CAD build for the part. Positions are in the model's coordinates, mm. Round coordinates to 2 decimals unless told otherwise and drop trailing zeros. Loops run counter-clockwise (first coordinate to the right, second up) from the corner with the lowest first, then second, coordinate; pieces in that order, holes last.
```python
from build123d import *
from build123d import SkipClean  # not in build123d's __all__

# Parameters (mm, degrees)
F0_W     = 14
F0_H     = 100
F0_R     = 1.64
F1_DEPTH = 1
F2_DEPTH = 10
F3_R     = 2
F4_DEPTH = 9.501


# Not quite as in the source:
# - after a boolean that leaves OpenCascade's solid faulty, fix() repairs it
# - a feature names something its author has since deleted; it is built from what else it names


with BuildPart() as f1:
    # F0 (on Front) → F1 (new body)
    with BuildSketch(Plane.XZ):
        Rectangle(F0_W, F0_H)
        with BuildLine():
            Line((-2.5, -44.5), (-2.5, -34.5))
            Line((-2.5, -34.5), (-0.8938540149, -34.5))
            ThreePointArc((-0.8938540149, -34.5), (-0.7822018331, -31.6835561779), (1.64, -33.125))
            ThreePointArc((1.64, -33.125), (1.4414438221, -33.9072018331), (0.8938540149, -34.5))
            Line((0.8938540149, -34.5), (2.5, -34.5))
            Line((2.5, -34.5), (2.5, -44.5))
            Line((2.5, -44.5), (0.8938540149, -44.5))
            ThreePointArc((0.8938540149, -44.5), (1.4414438221, -45.0927981669), (1.64, -45.875))
            ThreePointArc((1.64, -45.875), (-0.7822018331, -47.3164438221), (-0.8938540149, -44.5))
            Line((-0.8938540149, -44.5), (-2.5, -44.5))
        make_face(mode=Mode.SUBTRACT)
        Polygon((5, -21.096), (5, -29), (-5, -29), align=None, mode=Mode.SUBTRACT)
        Polygon((5, -19.096), (-5, -27), (-5, -11.192), align=None, mode=Mode.SUBTRACT)
        Polygon((5, -17.096), (-5, -9.192), (5, -1.288), align=None, mode=Mode.SUBTRACT)
        with Locations((-3.5, 45.167)):
            Circle(F0_R, mode=Mode.SUBTRACT)
        Polygon((-5, -7.19), (-5, 8.618), (5, 0.714), align=None, mode=Mode.SUBTRACT)
        Polygon((5, 18.522), (5, 2.714), (-5, 10.618), align=None, mode=Mode.SUBTRACT)
        Polygon((-5, 12.62), (-5, 28.428), (5, 20.524), align=None, mode=Mode.SUBTRACT)
        Polygon((5, 38.332), (5, 22.524), (-5, 30.428), align=None, mode=Mode.SUBTRACT)
        Polygon((5, 40.334), (-5, 32.43), (-5, 40.334), align=None, mode=Mode.SUBTRACT)
        with Locations((3.5, 45.167)):
            Circle(F0_R, mode=Mode.SUBTRACT)
        with BuildLine():
            Line((-0.8938540149, -34.5), (-2.5, -34.5))
            Line((-2.5, -34.5), (-2.5, -44.5))
            Line((-2.5, -44.5), (-0.8938540149, -44.5))
            ThreePointArc((-0.8938540149, -44.5), (0, -44.235), (0.8938540149, -44.5))
            Line((0.8938540149, -44.5), (2.5, -44.5))
            Line((2.5, -44.5), (2.5, -34.5))
            Line((2.5, -34.5), (0.8938540149, -34.5))
            ThreePointArc((0.8938540149, -34.5), (0, -34.765), (-0.8938540149, -34.5))
        make_face()
    extrude(amount=F1_DEPTH)

    # F0 (on Front) → F2 (join)
    with BuildSketch(Plane.XZ):
        with BuildLine():
            Line((-0.8938540149, -34.5), (-2.5, -34.5))
            Line((-2.5, -34.5), (-2.5, -44.5))
            Line((-2.5, -44.5), (-0.8938540149, -44.5))
            ThreePointArc((-0.8938540149, -44.5), (0, -44.235), (0.8938540149, -44.5))
            Line((0.8938540149, -44.5), (2.5, -44.5))
            Line((2.5, -44.5), (2.5, -34.5))
            Line((2.5, -34.5), (0.8938540149, -34.5))
            ThreePointArc((0.8938540149, -34.5), (0, -34.765), (-0.8938540149, -34.5))
        make_face()
    with SkipClean():  # cleaning this boolean's faces spoils the solid; the shape is the same uncleaned
        extrude(amount=-F2_DEPTH)

    # F3 (on face) → F4 (cut, through all)
    with BuildSketch(Plane.YZ.offset(2.5)):
        with BuildLine():
            Line((5, -44.5), (10, -44.5))
            Line((10, -44.5), (10, -39.5))
            ThreePointArc((10, -39.5), (8.5355339059, -43.0355339059), (5, -44.5))
        make_face()
        with Locations((5, -39.5)):
            Circle(F3_R)
        with BuildLine():
            ThreePointArc((5, -34.5), (8.5355339059, -35.9644660941), (10, -39.5))
            Line((10, -39.5), (10, -34.5))
            Line((10, -34.5), (5, -34.5))
        make_face()
    extrude(amount=-F4_DEPTH, mode=Mode.SUBTRACT)

    add(f1.part.fix(), mode=Mode.REPLACE)


solid = f1.part
```
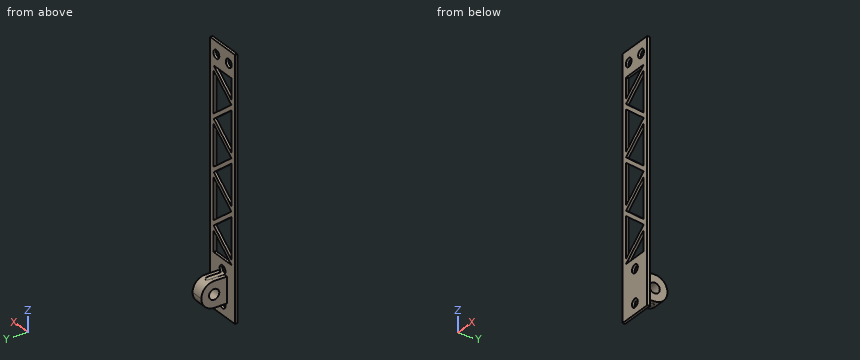
Item 1: Cut at B-B, the plane x = 0. State how many separate pieces and enclosed holes the cut face has, plus the area to 3 significant figures.
Answers follow:
separate pieces: 11
enclosed holes: 1
area: 112 mm2
Item 2: Flat gauge pins, fed straight in: P1, Ø0.8, axis at x = 1.5, y = 2.5, coming from the -Z side; P2, Ø4, axis at x = 0, z = -45.875, coming from the +Y side; P3, Ø4, axis at x = -3.5, z = 45.167, coming from the +Y side. Where does each tip first touch, or does it go through?
Answers follow:
P1: stops at z = -44.5
P2: stops at y = 7.42
P3: stops at y = 0
Item 3: Probe line 1 (Y direction, x = 6, z = 10.5); line 2 (Z direction, x = 0.25, y = 0.25); line 3 (X direction, y = 6, z = -42). List the from-to ranges inside material, lowest first.
Answers follow:
line 1: y = -1 to 0
line 2: z = -44.25 to -34.75
line 3: x = -2.5 to 2.5
Item 4: Cut at C-C, the plane y = 1. Give the cut face in (x, z) (3 decimals).
Answers follow:
outline: (-2.5, -44.5) - (-0.894, -44.5) arc R1.64 cw to (0.894, -44.5) - (2.5, -44.5) - (2.5, -34.5) - (0.894, -34.5) arc R1.64 cw to (-0.894, -34.5) - (-2.5, -34.5) - close
Item 5: Cut at A-A, the plane z = 9.5. Give the cut face in (x, y).
Answers follow:
outline: (-7, -1) - (-3.59, -1) - (-3.59, 0) - (-7, 0) - close; (5, -1) - (7, -1) - (7, 0) - (5, 0) - close
